Autodesk Fusion 360 part; units mm, degrees
sketch "Sketch1" plane through (0, 0, 0) normal (0, 0, 1) x (1, 0, 0)
  circle A0 centre (0, 0) radius 10.6
  line L0 (-33, 7.5) -> (-43, 7.5)
  arc A1 (-43, 7.5) -> (-43, -7.5) centre (-43, 0) ccw
  line L1 (-43, -7.5) -> (-33, -7.5)
  arc A2 (-33, -7.5) -> (-33, 7.5) centre (-33, 0) ccw
  line L2 (-25.5, 0) -> (-50.5, 0) construction
  line L3 (-20, 14.75) -> (-30, 14.75)
  arc A3 (-30, 14.75) -> (-30, 11.25) centre (-30, 13) ccw
  line L4 (-30, 11.25) -> (-20, 11.25)
  arc A4 (-20, 11.25) -> (-20, 14.75) centre (-20, 13) ccw
  line L5 (-18.25, 13) -> (-31.75, 13) construction
  line L6 (-43, 0) -> (-33, 0) construction
  line L7 (-30, 13) -> (-20, 13) construction
  line L8 (0, 0) -> (-73, 0) construction
  line L9 (-20, -14.75) -> (-30, -14.75)
  arc A5 (-30, -11.25) -> (-30, -14.75) centre (-30, -13) ccw
  line L10 (-30, -11.25) -> (-20, -11.25)
  arc A6 (-20, -14.75) -> (-20, -11.25) centre (-20, -13) ccw
  line L11 (-38, 0) -> (-38, 13) construction
  line L12 (-56, 14.75) -> (-46, 14.75)
  arc A7 (-46, 11.25) -> (-46, 14.75) centre (-46, 13) ccw
  line L13 (-46, 11.25) -> (-56, 11.25)
  arc A8 (-56, 14.75) -> (-56, 11.25) centre (-56, 13) ccw
  line L14 (-56, -14.75) -> (-46, -14.75)
  arc A9 (-56, -11.25) -> (-56, -14.75) centre (-56, -13) ccw
  line L15 (-46, -11.25) -> (-56, -11.25)
  arc A10 (-46, -14.75) -> (-46, -11.25) centre (-46, -13) ccw
  line L16 (-73, 30) -> (73, 30)
  line L17 (73, 30) -> (73, -30)
  line L18 (73, -30) -> (-73, -30)
  line L19 (-73, -30) -> (-73, 30)
  line L20 (-63, 20) -> (-13, 20) construction
  line L21 (-13, 20) -> (-13, -20) construction
  line L22 (-13, -20) -> (-63, -20) construction
  line L23 (-63, -20) -> (-63, 20) construction
  line L24 (0, 30) -> (0, -30) construction
  line L25 (63, 20) -> (13, 20)
  line L26 (63, -20) -> (63, 20)
  line L27 (13, -20) -> (63, -20)
  line L28 (13, 20) -> (13, -20)
  circle A11 centre (-66, 23) radius 2.6
  circle A12 centre (-66, -23) radius 2.6
  circle A13 centre (66, 23) radius 2.6
  circle A14 centre (66, -23) radius 2.6
  point P0 (-38, 0)
  point P1 (0, -30)
  point P2 (-63, 0)
  dimension "d1" = 21.2
  dimension "d2" = 10
  dimension "d3" = 15
  dimension "d4" = 20
  dimension "d5" = 26
  dimension "d6" = 3.5
  dimension "d7" = 26
  dimension "d12" = 7
  dimension "d13" = 7
  dimension "d14" = 7
  dimension "d15" = 10
  dimension "d16" = 10
  dimension "d17" = 5.2
  dimension "d18" = 7
  dimension "d19" = 7
extrude "Extrude1" add sketch "Sketch1" along normal blind 5
sketch "Sketch2" plane through (0, 0, 0) normal (0, 0, 1) x (1, 0, 0)
  circle A0 centre (0, 0) radius 11
  circle A1 centre (0, 0) radius 9.5
  dimension "d22" = 19
  dimension "d23" = 22
extrude "Extrude2" add sketch "Sketch2" along normal blind 1
fillet "Fillet1" radius 5 4 edges at (-73, 30, 2.5) (-73, -30, 2.5) (73, 30, 2.5) (73, -30, 2.5)
Could you check a few things on this model? Use its own coordinates, in mm. A direction names the side the tool comes from. Round coordinates to 2 decimals unless told otherwise and drop trailing zeros. Write each loop counter-clockwise with the first axis right and the second up, starting at its lowest first coordinate (ties: lowest second). Pieces come first, ordered by that corner, then holes. Notation, with made-up numbers: (58.25, -26.5) -> (114.25, -26.5) arc R13 ccw to (114.25, -10.5) -> close; hole circle Ø4 at (-24.5, 32.5). An arc over 180 degrees is marked (long way). Use a Markdown table: item, result.
1. If we section it at D-D (y = 13): List the corners of the cut face in (x, z) for me.
Answer key:
| item | result |
|---|---|
| outline | (-73, 0) -> (-57.75, 0) -> (-57.75, 5) -> (-73, 5) -> close; (-44.25, 0) -> (-31.75, 0) -> (-31.75, 5) -> (-44.25, 5) -> close; (-18.25, 0) -> (13, 0) -> (13, 5) -> (-18.25, 5) -> close; (63, 0) -> (73, 0) -> (73, 5) -> (63, 5) -> close |
2. Please list where these lines run through material, in increasing order: probe 1 along Y at (x, z) = (-66, 2.2); probe 2 along X at (y, z) = (15, 2.4); probe 3 along X at (y, z) = (-4.5, 0.2).
Answer key:
| item | result |
|---|---|
| probe 1 | y = -30 to -25.6, -20.4 to 20.4, 25.6 to 30 |
| probe 2 | x = -73 to 13, 63 to 73 |
| probe 3 | x = -73 to -49, -27 to -8.37, 8.37 to 13, 63 to 73 |
3. If we section it at C-C (x = -66): List the corners of the cut face in (y, z) for me.
Answer key:
| item | result |
|---|---|
| outline | (-30, 0) -> (-25.6, 0) -> (-25.6, 5) -> (-30, 5) -> close; (-20.4, 0) -> (20.4, 0) -> (20.4, 5) -> (-20.4, 5) -> close; (25.6, 0) -> (30, 0) -> (30, 5) -> (25.6, 5) -> close |
4. Which directions (+Z, -Z, +X, -X, +Y, -Y) give clear straight access to the entire face, cutting with the end or side of a thin tool? Please do faces 1 (the face through (-9, 4, 1)), 2 (the face through (-1, 30, 2)), 3 (the face through (-51, -11.25, 2)).
Answer key:
| item | result |
|---|---|
| face 1 | +Z |
| face 2 | +Z, -Z, +X, -X, +Y |
| face 3 | +Z, -Z |
5. If we section it at A-A (x = 41.5): List the corners of the cut face in (y, z) for me.
Answer key:
| item | result |
|---|---|
| outline | (-30, 0) -> (-20, 0) -> (-20, 5) -> (-30, 5) -> close; (20, 0) -> (30, 0) -> (30, 5) -> (20, 5) -> close |
6. For pin 1 Ø17 at (x, y) = (0, 0) entering from -Z, with a flat end and sliding along its axis, tell me the tip position at first contact or that it passes through.
Answer key:
| item | result |
|---|---|
| pin 1 | passes through |
7. We'd pull the mould along Y, two halves only. Please class faces 4 (the face through (4.38, 8.43, 0.49)), 5 (the face through (73, 0, 2)), 6 (the face through (72, 28, 3)): +Y half, -Y half, draft (parallel to the pull), parting line (faces both ways), or undercut.
Answer key:
| item | result |
|---|---|
| face 4 | undercut |
| face 5 | draft |
| face 6 | +Y half |
8. If we section it at B-B (y = -23): List the corners of the cut face in (x, z) for me, then the cut area to 3 significant figures.
Answer key:
| item | result |
|---|---|
| outline | (-73, 0) -> (-68.6, 0) -> (-68.6, 5) -> (-73, 5) -> close; (-63.4, 0) -> (63.4, 0) -> (63.4, 5) -> (-63.4, 5) -> close; (68.6, 0) -> (73, 0) -> (73, 5) -> (68.6, 5) -> close |
| area | 678 mm^2 |
